from build123d import *

# Parameters (mm, degrees)
SALIENTE_EXTRUIR1_DEPTH = 11.5
CORTAR_EXTRUIR1_START   = -2.4
CROQUIS2_R              = 2.1
CORTAR_EXTRUIR1_DEPTH   = 2.4
CROQUIS3_R              = 4.5
CORTAR_EXTRUIR2_DEPTH   = 0.5
CROQUIS4_R              = 3
CORTAR_EXTRUIR3_DEPTH   = 0.2


with BuildPart() as part:
    # Croquis1 → Saliente-Extruir1 (new body)
    with BuildSketch(Plane.XY):
        Polygon((-89.253382482, -13.336480186), (-89.253382482, 19.863519814), (-87.853382482, 19.863519814), (-87.853382482, 16.863519814), (-86.853382482, 16.863519814), (-86.853382482, 10.863519814), (-87.853382482, 10.863519814), (-87.853382482, -10.336480186), (-86.853382482, -10.336480186), (-86.853382482, -13.336480186), align=None)
    extrude(amount=SALIENTE_EXTRUIR1_DEPTH)

    # Croquis2 → Cortar-Extruir1 (cut)
    with BuildSketch(Plane(origin=(-86.853382482, 0, 0), x_dir=(0, 0, -1), z_dir=(1, 0, 0)).offset(CORTAR_EXTRUIR1_START)):
        with Locations((-5.75, 13.863519814)):
            Circle(CROQUIS2_R)
        with Locations((-5.75, -2.336480186)):
            Circle(CROQUIS2_R)
    extrude(amount=CORTAR_EXTRUIR1_DEPTH, mode=Mode.SUBTRACT)

    # Croquis3 → Cortar-Extruir2 (cut)
    with BuildSketch(Plane(origin=(-87.853382482, 0, 0), x_dir=(0, 0, -1), z_dir=(1, 0, 0))):
        with Locations((-5.75, -2.336480186)):
            Circle(CROQUIS3_R)
    extrude(amount=-CORTAR_EXTRUIR2_DEPTH, mode=Mode.SUBTRACT)

    # Croquis4 → Cortar-Extruir3 (cut)
    with BuildSketch(Plane.ZY.offset(89.253382482)):
        with Locations((5.75, 13.863519814)):
            Circle(CROQUIS4_R)
    extrude(amount=-CORTAR_EXTRUIR3_DEPTH, mode=Mode.SUBTRACT)


solid = part.part
Part model, mm, in its own coordinate system. A direction names the side the tool comes from. Coordinates: 2 decimals unless noted, no trailing zeros. Order: outer loops, then holes, each group sorted by start corner. A loop starts at its lowest first (then second) coordinate and runs counter-clockwise, first axis right, second up.
(1) Pin check, flat tips, straight feed: pin 1 Ø3 at (y, z) = (13, 5) entering from -X; pin 2 Ø2 at (y, z) = (14, 8.5) entering from -X; pin 3 Ø0.5 at (x, z) = (-87.5, 4) entering from +Y; pin 4 Ø1.5 at (y, z) = (18, 3) entering from +X. Stop position of each tip, or through.
Check sheet entries:
pin 1: stops at x = -89.05
pin 2: stops at x = -89.25
pin 3: stops at y = 16.86
pin 4: stops at x = -87.85
(2) Pull direction Y, two halves, no side cores. Call faces 4 (the face through (-89, 19.864, 6)), 5 (the face through (-87.853, 18, 6)), 6 (the face through (-88, -13.336, 6)), 7 (the face through (-87.969, 15.946, 6.023)): pulls with the +Y half, pulls with the -Y half, needs draft (parallel to the pull), parting line crosses it, or undercut.
Check sheet entries:
face 4: pulls with the +Y half
face 5: needs draft
face 6: pulls with the -Y half
face 7: undercut
(3) Probe L1, parallel to Y at x = -88, z = 5.75; L2, parallel to Y at x = -87.7, z = 2.75; L3, parallel to Y at x = -88.4, z = 5.75. List the from-to ranges inside material, lowest first.
Check sheet entries:
L1: y = -13.34 to -6.84, 2.16 to 11.76, 15.96 to 19.86
L2: y = -13.34 to -10.34, 10.86 to 16.86
L3: y = -13.34 to -4.44, -0.24 to 11.76, 15.96 to 19.86
(4) Slice it at B-B, the plane z = 7. Write the cut outline in (x, y).
Check sheet entries:
outline: (-89.25, -13.34) - (-86.85, -13.34) - (-86.85, -10.34) - (-87.85, -10.34) - (-87.85, -6.66) - (-88.35, -6.66) - (-88.35, -4.02) - (-89.25, -4.02) - close; (-89.25, -0.65) - (-88.35, -0.65) - (-88.35, 1.99) - (-87.85, 1.99) - (-87.85, 10.86) - (-86.85, 10.86) - (-86.85, 12.18) - (-89.05, 12.18) - (-89.05, 11.14) - (-89.25, 11.14) - close; (-89.25, 16.59) - (-89.05, 16.59) - (-89.05, 15.55) - (-86.85, 15.55) - (-86.85, 16.86) - (-87.85, 16.86) - (-87.85, 19.86) - (-89.25, 19.86) - close
(5) Tool access for faces 1 (the face through (-89.053, 16, 5)), 2 (the face through (-87.3, 10.864, 5.7)), 3 (the face through (-88.353, 0, 5)): list every direction of +Z, -Z, +X, -X, +Y, -Y with a clear straight run to the whole face (end or side of a thin tool).
Check sheet entries:
face 1: -X
face 2: +Z, -Z, +X
face 3: +X
(6) Slice it at D-D, the plane z = 9.25. Write the cut outline in (x, y), and give its area (3 significant figures).
Check sheet entries:
outline: (-89.25, -13.34) - (-86.85, -13.34) - (-86.85, -10.34) - (-87.85, -10.34) - (-87.85, -5.16) - (-88.35, -5.16) - (-88.35, 0.49) - (-87.85, 0.49) - (-87.85, 10.86) - (-86.85, 10.86) - (-86.85, 16.86) - (-87.85, 16.86) - (-87.85, 19.86) - (-89.25, 19.86) - close
area: 52.7 mm2
(7) Slice it at A-A, the plane x = -87.4. Write the cut outline in (y, z), and give its area (3 significant figures).
Check sheet entries:
outline: (-13.34, 0) - (-10.34, 0) - (-10.34, 11.5) - (-13.34, 11.5) - close; (10.86, 0) - (16.86, 0) - (16.86, 11.5) - (10.86, 11.5) - close; hole circle Ø4.2 at (13.86, 5.75)
area: 89.6 mm2
(8) Slice it at C-C, the plane y = 15.5. Write the cut outline in (x, z), and give its area (3 significant figures).
Check sheet entries:
outline: (-89.25, 0) - (-86.85, 0) - (-86.85, 4.43) - (-89.05, 4.43) - (-89.05, 3.24) - (-89.25, 3.24) - close; (-89.25, 8.26) - (-89.05, 8.26) - (-89.05, 7.07) - (-86.85, 7.07) - (-86.85, 11.5) - (-89.25, 11.5) - close
area: 20.8 mm2
